Geometry: final body of the model. Coordinates: model frame, mm. A direction names the side the tool comes from. Round coordinates to 2 decimals unless told otherwise and drop trailing zeros. Loops run counter-clockwise (first coordinate to the right, second up) from the corner with the lowest first, then second, coordinate; pieces in that order, holes last. Notation, with made-up numbers: (21.5, 81) - (53.5, 81) arc R20 ccw to (53.5, 99) - close; hole circle Ø1 at (-40, 51.5). An arc over 180 degrees is marked (long way). Answer as CSV lines item,"result".
from build123d import *

# Parameters (mm, degrees)
SKETCH_R           = 0.5
SKETCH_W           = 1.5
SKETCH_H           = 1
PAD_DEPTH          = 0.5
PAD_DEPTH_BACK     = 0.55
SKETCH001_W        = 4.919434
SKETCH001_H        = 5.037946
POCKET_DEPTH       = 1.05
POCKET_DEPTH_BACK  = 1.55
SKETCH006_W        = 1.496239
SKETCH006_H        = 0.320585
POCKET003_DEPTH    = 5
SKETCH002_R        = 0.51
SKETCH002_R_2      = 0.4
PAD001_DEPTH       = 1.5
SKETCH003_R        = 1
PAD002_DEPTH       = 0.2
SKETCH004_R        = 0.4
POCKET001_DEPTH    = 1
FILLET_R           = 0.1
SKETCH005_W        = 0.1
SKETCH005_H        = 1.784702
POCKET002_DEPTH    = 0.1
POLARPATTERN_COUNT = 6
PAD003_DEPTH       = 0.25


with BuildPart() as part:
    # Sketch → Pad (new body, two sides)
    with BuildSketch(Plane.XY) as pad_sk:
        with BuildLine():
            ThreePointArc((1.75, 0), (0, 1.75), (-1.75, 0))
            Line((-1.75, 0), (-1.75, -4.25))
            Line((-1.75, -4.25), (-1.75, -8))
            Line((-1.75, -8), (1.75, -8))
            Line((1.75, -8), (1.75, -4.25))
            Line((1.75, -4.25), (1.75, 0))
        make_face()
        Circle(SKETCH_R, mode=Mode.SUBTRACT)
        with Locations((0, -2.75)):
            Rectangle(SKETCH_W, SKETCH_H, mode=Mode.SUBTRACT)
    extrude(amount=PAD_DEPTH)
    extrude(pad_sk.sketch, amount=-PAD_DEPTH_BACK)

    # Sketch001 → Pocket (cut, two sides)
    with BuildSketch(Plane.XY) as pocket_sk:
        with Locations((-0.357018, -5.727314)):
            Rectangle(SKETCH001_W, SKETCH001_H)
    extrude(amount=-POCKET_DEPTH, mode=Mode.SUBTRACT)
    extrude(pocket_sk.sketch, amount=POCKET_DEPTH_BACK, mode=Mode.SUBTRACT)

    # Sketch006 → Pocket003 (cut)
    with BuildSketch(Plane.XY):
        with Locations((-0.005068, -3.405655)):
            Rectangle(SKETCH006_W, SKETCH006_H)
    extrude(amount=-POCKET003_DEPTH, mode=Mode.SUBTRACT)

    # Sketch002 → Pad001 (join)
    with BuildSketch(Plane.XY):
        Circle(SKETCH002_R)
        Circle(SKETCH002_R_2, mode=Mode.SUBTRACT)
    extrude(amount=PAD001_DEPTH)

    # Sketch003 → Pad002 (join)
    with BuildSketch(Plane.XY.offset(1.5)):
        Circle(SKETCH003_R)
    extrude(amount=PAD002_DEPTH)

    # Sketch004 → Pocket001 (cut)
    with BuildSketch(Plane.XY.offset(1.7)):
        Circle(SKETCH004_R)
    extrude(amount=-POCKET001_DEPTH, mode=Mode.SUBTRACT)

    # Fillet
    fillet_edges = [part.edges().sort_by_distance(p)[0] for p in [
        (-0.4, 0, 1.7),
        (-1, 0, 1.7),
    ]]
    fillet(fillet_edges, radius=FILLET_R)

    # Sketch005 → Pocket002 (cut)
    with BuildSketch(Plane.XY.offset(1.7)):
        with Locations((0, 0.892351)):
            Rectangle(SKETCH005_W, SKETCH005_H)
    pocket002 = extrude(amount=-POCKET002_DEPTH, mode=Mode.SUBTRACT)

    # PolarPattern: Pocket002 ×6 about axis
    polarpattern_axis = Axis((0, 0, 1.7), (0, 0, 1))
    for i in range(1, POLARPATTERN_COUNT):
        add(pocket002.rotate(polarpattern_axis, i * 360 / POLARPATTERN_COUNT), mode=Mode.SUBTRACT)

    # Sketch007 → Pad003 (join, symmetric)
    with BuildSketch(Plane(origin=(0, -2.75, -0.05), x_dir=(-1, 0, 0), z_dir=(0, -1, 0))):
        with BuildLine():
            Line((-1.75, -0.55), (1.75, -0.55))
            Line((1.75, -0.55), (1.75, -1.05))
            Line((0.5, -1.05), (1.75, -1.05))
            Line((0.5, -5.55), (0.5, -1.05))
            ThreePointArc((-0.5, -5.55), (0, -6.05), (0.5, -5.55))
            Line((-0.5, -1.05), (-0.5, -5.55))
            Line((-1.75, -1.05), (-0.5, -1.05))
            Line((-1.75, -1.05), (-1.75, -0.55))
        make_face()
    extrude(amount=PAD003_DEPTH, both=True)


with BuildPart() as part_1:
    # Body001 placement: moved
    add(part.part.moved(Location((-5, 0, 0))))


solid = part_1.part
(1) Access query for faces 1 (the face through (-5.75, -3, 0)), 2 (the face through (-5, -2.25, 0)), 3 (the face through (-5, -3, 3)). Directions: +Z, -Z, +X, -X, +Y, -Y. A direction counts if a zero-diameter tool reaches every point of the face in a straight line with its end or side. Return the directions, or none.
Findings below:
face 1,"-Z, -Y"
face 2,"+Z, -Z, -Y"
face 3,"+Z, +X, -X, -Y"
(2) Material intervals for line 1 along Z through (x, y) = (-5.1, 0.65); line 2 along X through (y, z) = (0, -0.15); line 3 along Y through (x, z) = (-5, -0.35), sorted ascending.
Findings below:
line 1,"-0.55 to 0.5, 1.5 to 1.7"
line 2,"-6.75 to -5.5, -4.5 to -3.25"
line 3,"-2.25 to -0.5, 0.5 to 1.75"
(3) Section C-C (x = -6.3). Output: boundary loops of the cut face in (y, z).
Findings below:
outline,"(-3.21, -0.55) - (1.17, -0.55) - (1.17, 0.5) - (-2.5, 0.5) - (-2.5, 1) - (-3, 1) - (-3, 0.5) - (-3.21, 0.5) - close"
(4) Section A-A (z = 0.75). Output: boundary loops of the cut face in (x, y).
Findings below:
outline,"(-6.75, -3) - (-3.25, -3) - (-3.25, -2.5) - (-6.75, -2.5) - close; circle Ø1.02 at (-5, 0); hole circle Ø0.8 at (-5, 0)"
(5) Section B-B (y = -2.15). Output: boundary loops of the cut face in (x, z), and give its area (4 significant figures).
Findings below:
outline,"(-6.75, -0.55) - (-3.25, -0.55) - (-3.25, 0.5) - (-6.75, 0.5) - close"
area,"3.675 mm2"
(6) Draft query along X for faces 4 (the face through (-6.75, -2, 0)), 5 (the face through (-5.4, -0.3, -0.3)), 6 (the face through (-5, -2.5, 3)). Return one class per face: pulls with the +X half, pulls with the -X half, needs draft (parallel to the pull), parting line crosses it, or undercut.
Findings below:
face 4,"pulls with the -X half"
face 5,"undercut"
face 6,"needs draft"
(7) Section D-D (z = 2.75). Output: boundary loops of the cut face in (x, y), and give its area (3 significant figures).
Findings below:
outline,"(-5.5, -3) - (-4.5, -3) - (-4.5, -2.5) - (-5.5, -2.5) - close"
area,"0.500 mm2"
(8) Pin query (flat end, axial travel): P1, Ø1, axis at x = -4.5, z = 3.5, coming from the +Y side; P2, Ø2, axis at y = 0.5, z = 2.5, coming from the -X side. Return the tip coordinate at first contact, or that it passes through.
Findings below:
P1,"y = -2.5"
P2,"x = -6"
